Print and shaded views of the part. All mm, measured from the part's lowest x, y and z. Coordinates: 2 decimals unless noted, no trailing zeros. Loops run counter-clockwise (first coordinate to the right, second up) from the corner with the lowest first, then second, coordinate; pieces in that order, holes last.
1) Saw through at B-B, the plane y = 1.75. Write the cut outline in (x, z) (1 decimal), and give its area (3 significant figures).
2) Saw through at D-D, the plane x = 15. Write the cut outline in (y, z) (3 decimals), and give its area (3 significant figures).
3) Pin check, flat tips, straight feed: pin 1 Ø1 at (x, z) = (9, 1.5) entering from +Y (1 decimal); pin 2 Ø1.5 at (x, y) = (15, 4.5) entering from +Z. Stop position of each tip, or through.
4) Wall check: line 1 along X through (y, z) = (6, 4) (3 decimals); line 2 along Y through (x, z) = (3.75, 2.25); line 3 along Z through (x, y) = (12.5, 1). Give the ranges that are in metal, low to high.
5) Saw through at A-A, the plane z = 6. Write the cut outline in (x, y) (1 decimal).
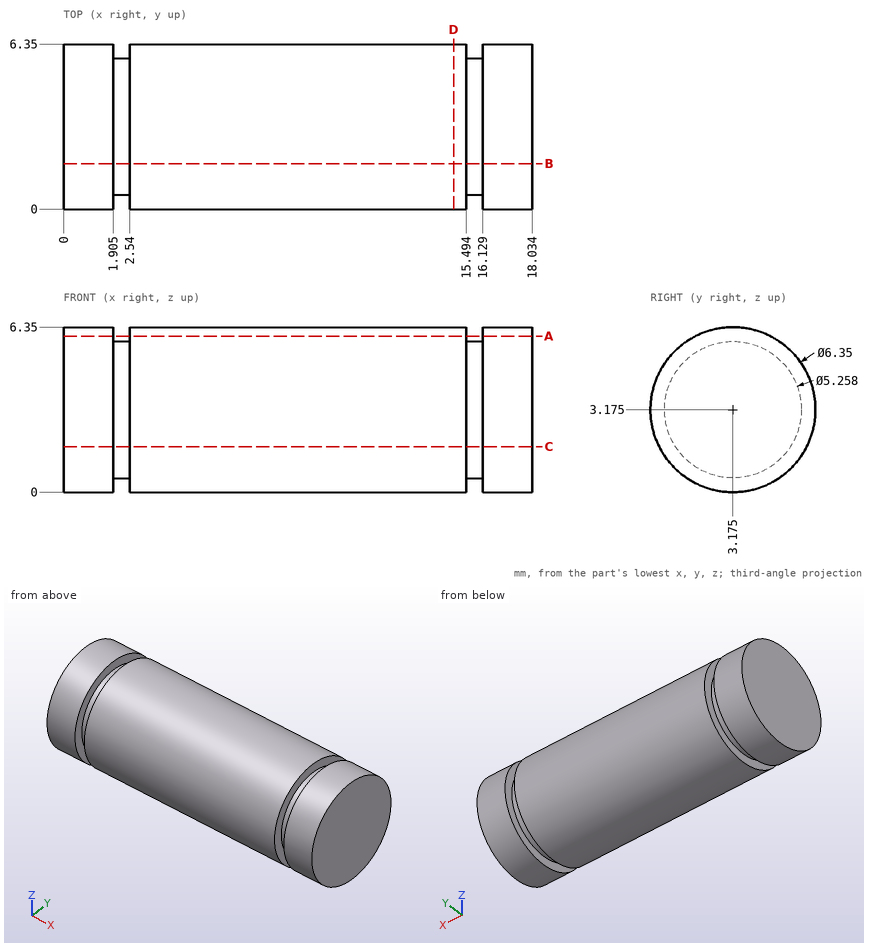
Data:
1. outline: (0, 0.3) - (1.9, 0.3) - (1.9, 1) - (2.5, 1) - (2.5, 0.3) - (15.5, 0.3) - (15.5, 1) - (16.1, 1) - (16.1, 0.3) - (18, 0.3) - (18, 6) - (16.1, 6) - (16.1, 5.4) - (15.5, 5.4) - (15.5, 6) - (2.5, 6) - (2.5, 5.4) - (1.9, 5.4) - (1.9, 6) - (0, 6) - close
1. area: 101 mm2
2. outline: circle Ø6.35 at (3.175, 3.175)
2. area: 31.7 mm2
3. pin 1: stops at y = 6.1
3. pin 2: stops at z = 6.3
4. line 1: x = 0 to 1.905, 2.54 to 15.494, 16.129 to 18.034
4. line 2: y = 0.14 to 6.21
4. line 3: z = 0.86 to 5.49
5. outline: (0, 1.7) - (1.9, 1.7) - (1.9, 4.6) - (0, 4.6) - close; (2.5, 1.7) - (15.5, 1.7) - (15.5, 4.6) - (2.5, 4.6) - close; (16.1, 1.7) - (18, 1.7) - (18, 4.6) - (16.1, 4.6) - close
